Autodesk Inventor part; units mm, degrees
ref_plane "YZ Plane" through (0, 0, 0) normal (1, 0, 0) x (0, 1, 0)
ref_plane "XZ Plane" through (0, 0, 0) normal (0, 1, 0) x (-1, 0, 0)
ref_plane "XY Plane" through (0, 0, 0) normal (0, 0, 1) x (1, 0, 0)
sketch "Sketch7" plane through (0, 0, 0) normal (0, 0, 1) x (1, 0, 0)
  circle A0 centre (-231.5775, 231.5775) radius 3.4
  line L0 (-231.5775, 203.2932) -> (-203.2932, 231.5775)
  line L1 (-203.2932, 231.5775) -> (-231.5775, 259.8617)
  line L2 (-231.5775, 259.8617) -> (-259.8617, 231.5775)
  line L3 (-259.8617, 231.5775) -> (-231.5775, 203.2932)
  line L4 (-231.5775, 203.2932) -> (-231.5775, 259.8617) construction
  line L5 (-203.2932, 231.5775) -> (-259.8617, 231.5775) construction
  line L6 (-231.5775, 203.2932) -> (-191.5775, 203.2932) construction
  arc A1 (289.9795, 47.2262) -> (285.9788, 67.3391) centre (0, 0) ccw construction
  arc A2 (295.9015, 48.1906) -> (291.8191, 68.7143) centre (0, 0) ccw
  arc A3 (284.0576, 46.2617) -> (280.1386, 65.9639) centre (0, 0) ccw
  arc A4 (284.0576, 46.2617) -> (295.9015, 48.1906) centre (289.9795, 47.2262) ccw
  arc A5 (291.8191, 68.7143) -> (280.1386, 65.9639) centre (285.9788, 67.3391) ccw
  line L7 (0, 0) -> (289.9795, 47.2262) construction
  line L8 (0, 0) -> (293.8, 0) construction
  line L9 (0, 0) -> (285.9788, 67.3391) construction
  circle A6 centre (0, 0) radius 307.5
  circle A7 centre (0, 0) radius 282.5
  line L10 (-203.2932, 231.5775) -> (-185.1143, 213.3986)
  line L11 (-231.5775, 203.2932) -> (-213.3986, 185.1143)
  line L12 (-307.5, 0) -> (0, 0)
  line L13 (0, 0) -> (307.5, 0)
  line L14 (-231.5775, -203.2932) -> (-259.8617, -231.5775)
  line L15 (-259.8617, -231.5775) -> (-231.5775, -259.8617)
  circle A8 centre (-231.5775, -231.5775) radius 3.4
  line L16 (-231.5775, -259.8617) -> (-203.2932, -231.5775)
  line L17 (-203.2932, -231.5775) -> (-231.5775, -203.2932)
  line L18 (-203.2932, -231.5775) -> (-185.1143, -213.3986)
  line L19 (-231.5775, -203.2932) -> (-213.3986, -185.1143)
  line L20 (203.2932, -231.5775) -> (231.5775, -259.8617)
  line L21 (231.5775, -259.8617) -> (259.8617, -231.5775)
  circle A9 centre (231.5775, -231.5775) radius 3.4
  line L22 (259.8617, -231.5775) -> (231.5775, -203.2932)
  line L23 (231.5775, -203.2932) -> (203.2932, -231.5775)
  line L24 (231.5775, -203.2932) -> (213.3986, -185.1143)
  line L25 (203.2932, -231.5775) -> (185.1143, -213.3986)
  line L26 (231.5775, 203.2932) -> (259.8617, 231.5775)
  line L27 (259.8617, 231.5775) -> (231.5775, 259.8617)
  circle A10 centre (231.5775, 231.5775) radius 3.4
  line L28 (231.5775, 259.8617) -> (203.2932, 231.5775)
  line L29 (203.2932, 231.5775) -> (231.5775, 203.2932)
  line L30 (203.2932, 231.5775) -> (185.1143, 213.3986)
  line L31 (231.5775, 203.2932) -> (213.3986, 185.1143)
  arc A11 (254.9356, 157.7589) -> (243.3099, 175.158) centre (0, 0) ccw
  arc A12 (243.3099, 175.158) -> (233.571, 168.1471) centre (238.4404, 171.6526) ccw
  arc A13 (244.7314, 151.4444) -> (233.571, 168.1471) centre (0, 0) ccw
  arc A14 (244.7314, 151.4444) -> (254.9356, 157.7589) centre (249.8335, 154.6017) ccw
  arc A15 (175.158, 243.3099) -> (157.7589, 254.9356) centre (0, 0) ccw
  arc A16 (157.7589, 254.9356) -> (151.4444, 244.7314) centre (154.6017, 249.8335) ccw
  arc A17 (168.1471, 233.571) -> (151.4444, 244.7314) centre (0, 0) ccw
  arc A18 (168.1471, 233.571) -> (175.158, 243.3099) centre (171.6526, 238.4404) ccw
  arc A19 (68.7143, 291.8191) -> (48.1906, 295.9015) centre (0, 0) ccw
  arc A20 (48.1906, 295.9015) -> (46.2617, 284.0576) centre (47.2262, 289.9795) ccw
  arc A21 (65.9639, 280.1386) -> (46.2617, 284.0576) centre (0, 0) ccw
  arc A22 (65.9639, 280.1386) -> (68.7143, 291.8191) centre (67.3391, 285.9788) ccw
  arc A23 (-48.1906, 295.9015) -> (-68.7143, 291.8191) centre (0, 0) ccw
  arc A24 (-68.7143, 291.8191) -> (-65.9639, 280.1386) centre (-67.3391, 285.9788) ccw
  arc A25 (-46.2617, 284.0576) -> (-65.9639, 280.1386) centre (0, 0) ccw
  arc A26 (-46.2617, 284.0576) -> (-48.1906, 295.9015) centre (-47.2262, 289.9795) ccw
  arc A27 (-157.7589, 254.9356) -> (-175.158, 243.3099) centre (0, 0) ccw
  arc A28 (-175.158, 243.3099) -> (-168.1471, 233.571) centre (-171.6526, 238.4404) ccw
  arc A29 (-151.4444, 244.7314) -> (-168.1471, 233.571) centre (0, 0) ccw
  arc A30 (-151.4444, 244.7314) -> (-157.7589, 254.9356) centre (-154.6017, 249.8335) ccw
  arc A31 (-243.3099, 175.158) -> (-254.9356, 157.7589) centre (0, 0) ccw
  arc A32 (-254.9356, 157.7589) -> (-244.7314, 151.4444) centre (-249.8335, 154.6017) ccw
  arc A33 (-233.571, 168.1471) -> (-244.7314, 151.4444) centre (0, 0) ccw
  arc A34 (-233.571, 168.1471) -> (-243.3099, 175.158) centre (-238.4404, 171.6526) ccw
  arc A35 (-291.8191, 68.7143) -> (-295.9015, 48.1906) centre (0, 0) ccw
  arc A36 (-295.9015, 48.1906) -> (-284.0576, 46.2617) centre (-289.9795, 47.2262) ccw
  arc A37 (-280.1386, 65.9639) -> (-284.0576, 46.2617) centre (0, 0) ccw
  arc A38 (-280.1386, 65.9639) -> (-291.8191, 68.7143) centre (-285.9788, 67.3391) ccw
  arc A39 (-295.9015, -48.1906) -> (-291.8191, -68.7143) centre (0, 0) ccw
  arc A40 (-291.8191, -68.7143) -> (-280.1386, -65.9639) centre (-285.9788, -67.3391) ccw
  arc A41 (-284.0576, -46.2617) -> (-280.1386, -65.9639) centre (0, 0) ccw
  arc A42 (-284.0576, -46.2617) -> (-295.9015, -48.1906) centre (-289.9795, -47.2262) ccw
  arc A43 (-254.9356, -157.7589) -> (-243.3099, -175.158) centre (0, 0) ccw
  arc A44 (-243.3099, -175.158) -> (-233.571, -168.1471) centre (-238.4404, -171.6526) ccw
  arc A45 (-244.7314, -151.4444) -> (-233.571, -168.1471) centre (0, 0) ccw
  arc A46 (-244.7314, -151.4444) -> (-254.9356, -157.7589) centre (-249.8335, -154.6017) ccw
  arc A47 (-175.158, -243.3099) -> (-157.7589, -254.9356) centre (0, 0) ccw
  arc A48 (-157.7589, -254.9356) -> (-151.4444, -244.7314) centre (-154.6017, -249.8335) ccw
  arc A49 (-168.1471, -233.571) -> (-151.4444, -244.7314) centre (0, 0) ccw
  arc A50 (-168.1471, -233.571) -> (-175.158, -243.3099) centre (-171.6526, -238.4404) ccw
  arc A51 (-68.7143, -291.8191) -> (-48.1906, -295.9015) centre (0, 0) ccw
  arc A52 (-48.1906, -295.9015) -> (-46.2617, -284.0576) centre (-47.2262, -289.9795) ccw
  arc A53 (-65.9639, -280.1386) -> (-46.2617, -284.0576) centre (0, 0) ccw
  arc A54 (-65.9639, -280.1386) -> (-68.7143, -291.8191) centre (-67.3391, -285.9788) ccw
  arc A55 (48.1906, -295.9015) -> (68.7143, -291.8191) centre (0, 0) ccw
  arc A56 (68.7143, -291.8191) -> (65.9639, -280.1386) centre (67.3391, -285.9788) ccw
  arc A57 (46.2617, -284.0576) -> (65.9639, -280.1386) centre (0, 0) ccw
  arc A58 (46.2617, -284.0576) -> (48.1906, -295.9015) centre (47.2262, -289.9795) ccw
  arc A59 (157.7589, -254.9356) -> (175.158, -243.3099) centre (0, 0) ccw
  arc A60 (175.158, -243.3099) -> (168.1471, -233.571) centre (171.6526, -238.4404) ccw
  arc A61 (151.4444, -244.7314) -> (168.1471, -233.571) centre (0, 0) ccw
  arc A62 (151.4444, -244.7314) -> (157.7589, -254.9356) centre (154.6017, -249.8335) ccw
  arc A63 (243.3099, -175.158) -> (254.9356, -157.7589) centre (0, 0) ccw
  arc A64 (254.9356, -157.7589) -> (244.7314, -151.4444) centre (249.8335, -154.6017) ccw
  arc A65 (233.571, -168.1471) -> (244.7314, -151.4444) centre (0, 0) ccw
  arc A66 (233.571, -168.1471) -> (243.3099, -175.158) centre (238.4404, -171.6526) ccw
  arc A67 (291.8191, -68.7143) -> (295.9015, -48.1906) centre (0, 0) ccw
  arc A68 (295.9015, -48.1906) -> (284.0576, -46.2617) centre (289.9795, -47.2262) ccw
  arc A69 (280.1386, -65.9639) -> (284.0576, -46.2617) centre (0, 0) ccw
  arc A70 (280.1386, -65.9639) -> (291.8191, -68.7143) centre (285.9788, -67.3391) ccw
  point P0 (-202.8328, 231.1171)
  point P1 (-231.1171, 202.8328)
  point P2 (-282.5, 0)
  point P3 (282.5, 0)
  point P4 (231.1171, 202.8328)
  point P5 (202.8328, 231.1171)
  dimension "d131" = 6.8
  dimension "d132" = 231.5775
  dimension "d133" = 231.5775
  dimension "d135" = 45
  dimension "d137" = 40
  dimension "d138" = 40
  dimension "d144" = 293.8
  dimension "d145" = 9.25
  dimension "d146" = 4
  dimension "d147" = 12
  dimension "d148" = 615
  dimension "d149" = 565
  dimension "d152" = 360
  dimension "d156" = 360
extrude "Extrusion11" add sketch "Sketch7" against normal blind 10 contours L3 L2 L1 L0 | L0 A6 L11 | L0 L10 A6 | A6 L10 A7 L11 | L11 A7 L12 A6 | A6 L30 A7 L10 | L30 L29 A6 | A6 L31 A7 L30 | L29 L31 A6 | L29 L28 L27 L26 | A6 L13 A7 L31
sketch "Sketch8" plane through (-307.5, 0, 0) normal (0, -1, 0) x (1, 0, 0)
  line L0 (25, 0) -> (590, 0)
  line L1 (25, 0) -> (-14, 0)
  line L2 (-14, 0) -> (-14, -10)
  line L3 (-14, -10) -> (25, -10)
  line L4 (25, -10) -> (25, 0)
  circle A0 centre (-7, -5) radius 3
  line L5 (590, 0) -> (629, 0)
  line L6 (629, 0) -> (629, -10)
  line L7 (629, -10) -> (590, -10)
  line L8 (590, -10) -> (590, 0)
  circle A1 centre (622, -5) radius 3
  dimension "d160" = 39
  dimension "d161" = 10
  dimension "d162" = 6
  dimension "d163" = 5
  dimension "d164" = 7
  dimension "d165" = 39
  dimension "d166" = 10
  dimension "d167" = 6
  dimension "d168" = 7
  dimension "d169" = 5
extrude "Extrusion12" add sketch "Sketch8" against normal blind 10
fillet "Fillet4" radius 4 8 edges at (-231.1171, 202.8328, -5) (-259.8617, 231.5775, -5) (-202.8328, 231.1171, -5) (-231.5775, 259.8617, -5) (231.5775, 259.8617, -5) (259.8617, 231.5775, -5) (202.8328, 231.1171, -5) (231.1171, 202.8328, -5)
equation "\"bar_screw_hole_diam\" = 6.8"
equation "\"foot_length\" = 14"
equation "\"tube_rim_diam\" = 605"
equation "\"tube_inner_diam\" = 541"
equation "\"tube_outer_diam\" = 561"
equation "\"ring_delta\" = 2"
equation "\"bar_delta\" = 5"
equation "\"bar_circle_diam\" = 655"
equation "\"ring_inner_diam\" = 565"
equation "\"ring_outer_diam\" = 615"
equation "\"slot_angle\" = 9.25deg"
equation "\"slot_diam\" = 12"
equation "\"slots_circle_diam\" = 587.6"
equation "\"foot_screw_diam\" = 6"
equation "\"bar_fillet\" = 4"
properties part number "half_ring_1" material "Aluminum 6061"
Input: part model. Units: mm. Frame: model coordinates. A direction names the side the tool comes from. Round coordinates to 2 decimals unless told otherwise and drop trailing zeros. Write each loop counter-clockwise with the first axis right and the second up, starting at its lowest first coordinate (ties: lowest second). Pieces come first, ordered by that corner, then holes.
1) Draft query along Y for faces 1 (the flat face through (-216.945, 245.229, -4.93)), 2 (the flat face through (-2, 291, -10)), 3 (the cylindrical face through (287.17, 109.95, -4.93)). Return one class per face: pulls with the +Y half, pulls with the -Y half, needs draft (parallel to the pull), parting line crosses it, or undercut.
2) Cut plane C-C (x = 0). Return the cut outline in (y, z), then the cut area to 3 significant figures.
3) Cut plane B-B (z = -5). Count the separate pieces of the cut face and the enclosed holes in it, then the cut area to 3 significant figures.
4) Cut plane A-A (y = 24). Return the cut outline in (x, z).
5) Cut plane D-D (x = -215). Return the cut outline in (y, z).
6) Contact query for flat-ended pins moving along their axis: P1, Ø2, axis at x = 223.5, z = -6, coming from the -Y side; P2, Ø1.5, axis at x = 125, z = -9, coming from the -Y side; P3, Ø1, axis at y = 77, z = -4.5, coming from the +X side. Output: stop coordinate, or through.
7) Ray query, L1, parallel to X at y = 172, z = -2.5; L2, parallel to X at y = 244.5, z = -5.75; L3, parallel to Z at x = -314.5, y = 2.75. Return the intervals inside material, ascending.
8) Reachability of faces 4 (the cylindrical face through (-166.438, 249.356, -4.93)), 5 (the flat face through (217.271, 245.555, -4.93)), 6 (the flat face through (-245.555, 217.271, -4.93)), 7 (the flat face through (245.88, 245.56, -4.93)), 8 (the flat face through (245.229, 216.945, -4.93)) from +Z, -Z, +X, -X, +Y, -Y: full face, straight path, thin tool, end or side. Return the list, or none.
Geometry says:
1. face 1: pulls with the +Y half
1. face 2: needs draft
1. face 3: undercut
2. outline: (282.5, -10) - (307.5, -10) - (307.5, 0) - (282.5, 0) - close
2. area: 250 mm2
3. separate pieces: 3
3. enclosed holes: 10
3. area: 23,600 mm2
4. outline: (-306.56, -10) - (-281.48, -10) - (-281.48, 0) - (-306.56, 0) - close; (281.48, -10) - (306.56, -10) - (306.56, 0) - (281.48, 0) - close
5. outline: (183.25, -10) - (243.28, -10) - (243.28, 0) - (183.25, 0) - close
6. P1: stops at y = 171.48
6. P2: stops at y = 252.97
6. P3: stops at x = 297.83
7. L1: x = -254.9 to -245.55, -232.45 to -224.1, 224.1 to 232.45, 245.55 to 254.9
7. L2: x = -246.94 to -216.22, -186.48 to -173.49, -151.82 to -141.51, 141.51 to 151.82, 173.49 to 186.48, 216.22 to 246.94
7. L3: z = -10 to -8, -2 to 0
8. face 4: +Z, -Z
8. face 5: +Z, -Z, +Y
8. face 6: +Z, -Z, -X
8. face 7: +Z, -Z, +X, +Y
8. face 8: +Z, -Z, +X
